Verification items for the finished model (mm, model axes). A direction names the side the tool comes from. Coordinates: 2 decimals unless noted, no trailing zeros. Order: outer loops, then holes, each group sorted by start corner. A loop starts at its lowest first (then second) coordinate and runs counter-clockwise, first axis right, second up. Notation, with made-up numbers: M 73,36 L 84,36 A11 cw 84,44 Z; hole C 19.5,64 d3. An arc over 180 degrees is marked long. Use one line per item in the form item = value. Start each with the question number.
```python
from build123d import *

# Parameters (mm, degrees)
SKETCH1_R           = 35
BOSS_EXTRUDE1_DEPTH = 2
SKETCH2_R           = 24
SKETCH2_R_2         = 21
BOSS_EXTRUDE2_DEPTH = 14
SKETCH3_R           = 21
CUT_EXTRUDE1_DEPTH  = 10
CUT_EXTRUDE2_REACH  = 18
SKETCH4_R           = 1.5
SKETCH5_R           = 21
SKETCH5_R_2         = 18
BOSS_EXTRUDE3_DEPTH = 2


with BuildPart() as part:
    # Sketch1 → Boss-Extrude1 (new body)
    with BuildSketch(Plane.XY):
        Circle(SKETCH1_R)
    extrude(amount=BOSS_EXTRUDE1_DEPTH)

    # Sketch2 → Boss-Extrude2 (add)
    with BuildSketch(Plane.XY.offset(2)):
        Circle(SKETCH2_R)
        Circle(SKETCH2_R_2, mode=Mode.SUBTRACT)
    extrude(amount=BOSS_EXTRUDE2_DEPTH)

    # Sketch3 → Cut-Extrude1 (cut)
    with BuildSketch(Plane.XY.offset(2)):
        Circle(SKETCH3_R)
    extrude(amount=-CUT_EXTRUDE1_DEPTH, mode=Mode.SUBTRACT)

    # Sketch4 → Cut-Extrude2 (cut, up to next)
    with BuildSketch(Plane(origin=(0, 0, 0), x_dir=(-1, 0, 0), z_dir=(0, 0, -1)), mode=Mode.PRIVATE) as cut_extrude2_sk1:
        with Locations((29, 0)):
            Circle(SKETCH4_R)
    cut_extrude2_tool1 = extrude(cut_extrude2_sk1.sketch, amount=-CUT_EXTRUDE2_REACH, mode=Mode.PRIVATE) & part.part
    add(cut_extrude2_tool1.solids().sort_by_distance((-29, 0, 0))[0], mode=Mode.SUBTRACT)
    # Sketch4 → Cut-Extrude2 (cut, up to next)
    with BuildSketch(Plane(origin=(0, 0, 0), x_dir=(-1, 0, 0), z_dir=(0, 0, -1)), mode=Mode.PRIVATE) as cut_extrude2_sk2:
        with Locations((0, -29)):
            Circle(SKETCH4_R)
    cut_extrude2_tool2 = extrude(cut_extrude2_sk2.sketch, amount=-CUT_EXTRUDE2_REACH, mode=Mode.PRIVATE) & part.part
    add(cut_extrude2_tool2.solids().sort_by_distance((0, -29, 0))[0], mode=Mode.SUBTRACT)
    # Sketch4 → Cut-Extrude2 (cut, up to next)
    with BuildSketch(Plane(origin=(0, 0, 0), x_dir=(-1, 0, 0), z_dir=(0, 0, -1)), mode=Mode.PRIVATE) as cut_extrude2_sk3:
        with Locations((-29, 0)):
            Circle(SKETCH4_R)
    cut_extrude2_tool3 = extrude(cut_extrude2_sk3.sketch, amount=-CUT_EXTRUDE2_REACH, mode=Mode.PRIVATE) & part.part
    add(cut_extrude2_tool3.solids().sort_by_distance((29, 0, 0))[0], mode=Mode.SUBTRACT)
    # Sketch4 → Cut-Extrude2 (cut, up to next)
    with BuildSketch(Plane(origin=(0, 0, 0), x_dir=(-1, 0, 0), z_dir=(0, 0, -1)), mode=Mode.PRIVATE) as cut_extrude2_sk4:
        with Locations((0, 29)):
            Circle(SKETCH4_R)
    cut_extrude2_tool4 = extrude(cut_extrude2_sk4.sketch, amount=-CUT_EXTRUDE2_REACH, mode=Mode.PRIVATE) & part.part
    add(cut_extrude2_tool4.solids().sort_by_distance((0, 29, 0))[0], mode=Mode.SUBTRACT)

    # Sketch5 → Boss-Extrude3 (add)
    with BuildSketch(Plane(origin=(0, 0, 0), x_dir=(-1, 0, 0), z_dir=(0, 0, -1))):
        Circle(SKETCH5_R)
        Circle(SKETCH5_R_2, mode=Mode.SUBTRACT)
    extrude(amount=-BOSS_EXTRUDE3_DEPTH)


solid = part.part
```
1. Cross-section at C-C on y = -29. Enter the section's corners in (x, z), and give its area (3 significant figures).
2. Release check for a two-part mould opening along X. For faces 3 (the cylindrical face through (30.5, 0.07, 0.99)), 4 (the cylindrical face through (2.343, 17.847, 0.986)), 5 (the flat face through (-15, -15, 0)), 6 (the cylindrical face through (-28, -21, 1)) record: pulls with the +X half, pulls with the -X half, needs draft (parallel to the pull), parting line crosses it, or undercut.
3. Material ranges on line 1 along Y through (x, z) = (0, 1.05); line 2 along Z through (x, y) = (13.5, 22); line 3 along Y through (x, z) = (-29, 0.6), recorded low to high.
4. Cross-section at A-A on x = 0. Enter the section's corners in (y, z), and give its area (3 significant figures).
5. Depth check by flat-ended pin: P1, Ø21, axis at x = -6, y = -1.5, coming from the +Z side; P2, Ø1.5, axis at x = 22.5, y = 15.5, coming from the +Z side; P3, Ø4, axis at y = 12, z = 4.5, coming from the -X side; P4, Ø3, axis at y = -10.5, z = 14, coming from the +X side. Enter the tip coordinate at first touch or a pass-through.
6. Tool access check on faces 1 (the cylindrical face through (0.195, -27.513, 0.986)), 2 (the flat face through (9, 16, 2)). Record the directions out of +Z, -Z, +X, -X, +Y, -Y that give a thin tool (end or side, any length) a straight path to the whole face; none if there is none.
7. Cross-section at D-D on z = 4.25. Enter the section's corners in (x, y).
Final values:
q1.outline = M -19.6,0 L -1.5,0 L -1.5,2 L -19.6,2 Z; M 1.5,0 L 19.6,0 L 19.6,2 L 1.5,2 Z
q1.area = 72.4 mm2
q2.face_3 = undercut
q2.face_4 = undercut
q2.face_5 = needs draft
q2.face_6 = parting line crosses it
q3.line_1 = -35 to -30.5, -27.5 to -18, 18 to 27.5, 30.5 to 35
q3.line_2 = 0 to 2
q3.line_3 = -19.6 to -1.5, 1.5 to 19.6
q4.outline = M -35,0 L -30.5,0 L -30.5,2 L -35,2 Z; M -27.5,0 L -18,0 L -18,2 L -21,2 L -21,16 L -24,16 L -24,2 L -27.5,2 Z; M 18,0 L 27.5,0 L 27.5,2 L 24,2 L 24,16 L 21,16 L 21,2 L 18,2 Z; M 30.5,0 L 35,0 L 35,2 L 30.5,2 Z
q4.area = 140 mm2
q5.P1 = through
q5.P2 = 2
q5.P3 = -21.82
q5.P4 = 22.25
q6.face_1 = +Z, -Z
q6.face_2 = +Z
q7.outline = C 0,0 d48; hole C 0,0 d42
